Read the model definition and answer for the solid it produces. Units are mm, in the model's axes. Face numbers are marked on the shaded views. Give positions to 0.01 mm unless a question says otherwise; leave off trailing zeros. Loops run counter-clockwise (first coordinate to the right, second up) from the corner with the lowest first, then second, coordinate; pieces in that order, holes last. Notation, with made-up numbers: (19, -38.75) - (78, -38.75) arc R16 cw to (78, -10.75) - close; hole circle Ø1 at (82.25, 79.25). An arc over 180 degrees is marked (long way). Write each question's results on one line, items separated by ' | '. Start each with the question number.
Q1. The part is cut by section C-C, the plane y = 14.5. Write down the section's boundary in (x, z).
Q2. Given pin 1 (3 mm diameter, centred on x = 47, y = -36.5, fed in from +Z), flat-ended and moving along its own axis, determine where the tip first touches the part or whether it passes through.
Q3. Find the intervals of material crossed by line 1 (X direction, y = -77, z = 34); line 2 (X direction, y = -2.5, z = 132); line 3 (Y direction, x = 47, z = 134.5), in increasing order. Write a range as from..to.
Q4. The part is cut by section D-D, the plane z = 34. Write down the section's boundary in (x, y).
Q5. The part is cut by section B-B, the plane z = 154.5. Write down the section's boundary in (x, y).
Q6. The part is cut by section A-A, the plane x = 0. Write down the section's boundary in (y, z).
Q7. Determine the mould class of the marked faces 1, 2, 3 and 4 for opening direction Y: +Y half, -Y half, draft (parallel to the pull), parting line (faces both ways), or undercut.
```python
from build123d import *

# Parameters (mm, degrees)
CROQUIS1_W              = 157.6
CROQUIS1_H              = 157.1
CROQUIS1_W_2            = 149
CROQUIS1_H_2            = 148.5
SALIENTE_EXTRUIR1_DEPTH = 204.5
CROQUIS2_W              = 4
CROQUIS2_H              = 157.1
SALIENTE_EXTRUIR2_DEPTH = 149
CROQUIS3_R              = 11
CORTAR_EXTRUIR1_DEPTH   = 4.3


with BuildPart() as part:
    # Croquis1 → Saliente-Extruir1 (new body)
    with BuildSketch(Plane.XY):
        Rectangle(CROQUIS1_W, CROQUIS1_H)
        Rectangle(CROQUIS1_W_2, CROQUIS1_H_2, mode=Mode.SUBTRACT)
    extrude(amount=SALIENTE_EXTRUIR1_DEPTH)

    # Croquis2 → Saliente-Extruir2 (add)
    with BuildSketch(Plane(origin=(-74.5, 0, 0), x_dir=(0, 0, -1), z_dir=(1, 0, 0))):
        with Locations((-2, 0)):
            Rectangle(CROQUIS2_W, CROQUIS2_H)
    extrude(amount=SALIENTE_EXTRUIR2_DEPTH)

    # Croquis3 → Cortar-Extruir1 (cut)
    with BuildSketch(Plane.XZ.offset(78.55)):
        with Locations(Location((0, 34, 0), (0, 0, 270))):
            Circle(CROQUIS3_R)
    extrude(amount=-CORTAR_EXTRUIR1_DEPTH, mode=Mode.SUBTRACT)


solid = part.part
```
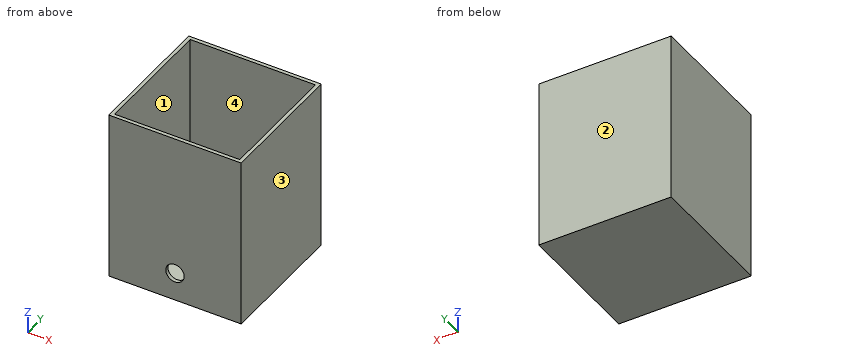
Check sheet entries:
1) outline: (-78.8, 0) - (78.8, 0) - (78.8, 204.5) - (74.5, 204.5) - (74.5, 4) - (-74.5, 4) - (-74.5, 204.5) - (-78.8, 204.5) - close
2) pin 1: stops at z = 4
3) line 1: x = -78.8..-11, 11..78.8 | line 2: x = -78.8..-74.5, 74.5..78.8 | line 3: y = -78.55..-74.25, 74.25..78.55
4) outline: (-78.8, -78.55) - (-11, -78.55) - (-11, -74.25) - (-74.5, -74.25) - (-74.5, 74.25) - (74.5, 74.25) - (74.5, -74.25) - (11, -74.25) - (11, -78.55) - (78.8, -78.55) - (78.8, 78.55) - (-78.8, 78.55) - close
5) outline: (-78.8, -78.55) - (78.8, -78.55) - (78.8, 78.55) - (-78.8, 78.55) - close; hole (-74.5, -74.25) - (74.5, -74.25) - (74.5, 74.25) - (-74.5, 74.25) - close
6) outline: (-78.55, 0) - (78.55, 0) - (78.55, 204.5) - (74.25, 204.5) - (74.25, 4) - (-74.25, 4) - (-74.25, 23) - (-78.55, 23) - close; (-78.55, 45) - (-74.25, 45) - (-74.25, 204.5) - (-78.55, 204.5) - close
7) face 1: undercut | face 2: +Y half | face 3: draft | face 4: undercut
